Part model, mm, in its own coordinate system. A direction names the side the tool comes from. Round coordinates to 2 decimals unless told otherwise and drop trailing zeros. Write each loop counter-clockwise with the first axis right and the second up, starting at its lowest first coordinate (ties: lowest second). Pieces come first, ordered by that corner, then holes. Notation, with made-up numbers: M -31,74 L 26,74 A16 ccw 26,83 Z; hole C 76.5,63 d6. An arc over 180 degrees is marked long. Answer as a JSON object with one key per item and string values. Group by question number.
1. Band-saw the part on A-A, the plane x = 6.75. Write the cut outline in (y, z), plus the area to 3 significant figures.
2. Which spindle directions (+Z, -Z, +X, -X, +Y, -Y) get a long thin tool onto all of the face, cutting with end or side? Do faces 4 (the face through (0, 5, -15)), 5 (the face through (0, 7, 0)). Say none if no direction does.
3. Band-saw the part on B-B, the plane y = 2.75. Write the cut outline in (x, z).
4. Two-plate mould, pull along Z, no slides. Class faces 1 (the face through (0, 5, 15)), 2 (the face through (0, 3, -3.5)), 3 (the face through (-15, 5, 0)): +Z half, -Z half, draft (parallel to the pull), parting line (faces both ways), or undercut.
5. Band-saw the part on C-C, the plane z = -2.75. Write the cut outline in (x, y).
6. Drill centre lines: line 1 (X direction, y = 4.75, z = -1.25); line 2 (Z direction, x = 4.5, y = 1.5); line 3 (Y direction, x = -4.25, z = -1.5). Where is each one in solid material? Low to high. Write a range as from..to.
7. Drop a flat-ended pin along its axis: pin 1 (5.5 mm diameter, centred on x = 5, z = -1, fed in from -Y). Give the stop position or say it passes through.
from build123d import *

# Parameters (mm, degrees)
SKETCH1_W           = 30
SKETCH1_H           = 30
SKETCH1_W_2         = 23
SKETCH1_H_2         = 7
BOSS_EXTRUDE1_DEPTH = 10
BOSS_EXTRUDE2_START = 7
SKETCH1_2_W         = 23
SKETCH1_2_H         = 7
BOSS_EXTRUDE2_DEPTH = 3


with BuildPart() as part:
    # Sketch1 → Boss-Extrude1 (new body)
    with BuildSketch(Plane(origin=(0, 0, 0), x_dir=(1, 0, 0), z_dir=(0, 1, 0))):
        Rectangle(SKETCH1_W, SKETCH1_H)
        Rectangle(SKETCH1_W_2, SKETCH1_H_2, mode=Mode.SUBTRACT)
    extrude(amount=BOSS_EXTRUDE1_DEPTH)

    # Sketch1<2> → Boss-Extrude2 (add)
    with BuildSketch(Plane(origin=(0, 0, 0), x_dir=(1, 0, 0), z_dir=(0, 1, 0)).offset(BOSS_EXTRUDE2_START)):
        Rectangle(SKETCH1_2_W, SKETCH1_2_H)
    extrude(amount=BOSS_EXTRUDE2_DEPTH)


solid = part.part
Worked answers:
{
 "1": {"outline": "M 0,-15 L 10,-15 L 10,15 L 0,15 L 0,3.5 L 7,3.5 L 7,-3.5 L 0,-3.5 Z", "area": "251 mm^2"},
 "2": {"face 4": "-Z, +X, -X, +Y, -Y", "face 5": "-Y"},
 "3": {"outline": "M -15,-15 L 15,-15 L 15,15 L -15,15 Z; hole M -11.5,-3.5 L 11.5,-3.5 L 11.5,3.5 L -11.5,3.5 Z"},
 "4": {"face 1": "+Z half", "face 2": "undercut", "face 3": "draft"},
 "5": {"outline": "M -15,0 L -11.5,0 L -11.5,7 L 11.5,7 L 11.5,0 L 15,0 L 15,10 L -15,10 Z"},
 "6": {"line 1": "x = -15..-11.5, 11.5..15", "line 2": "z = -15..-3.5, 3.5..15", "line 3": "y = 7..10"},
 "7": {"pin 1": "stops at y = 0"}
}
